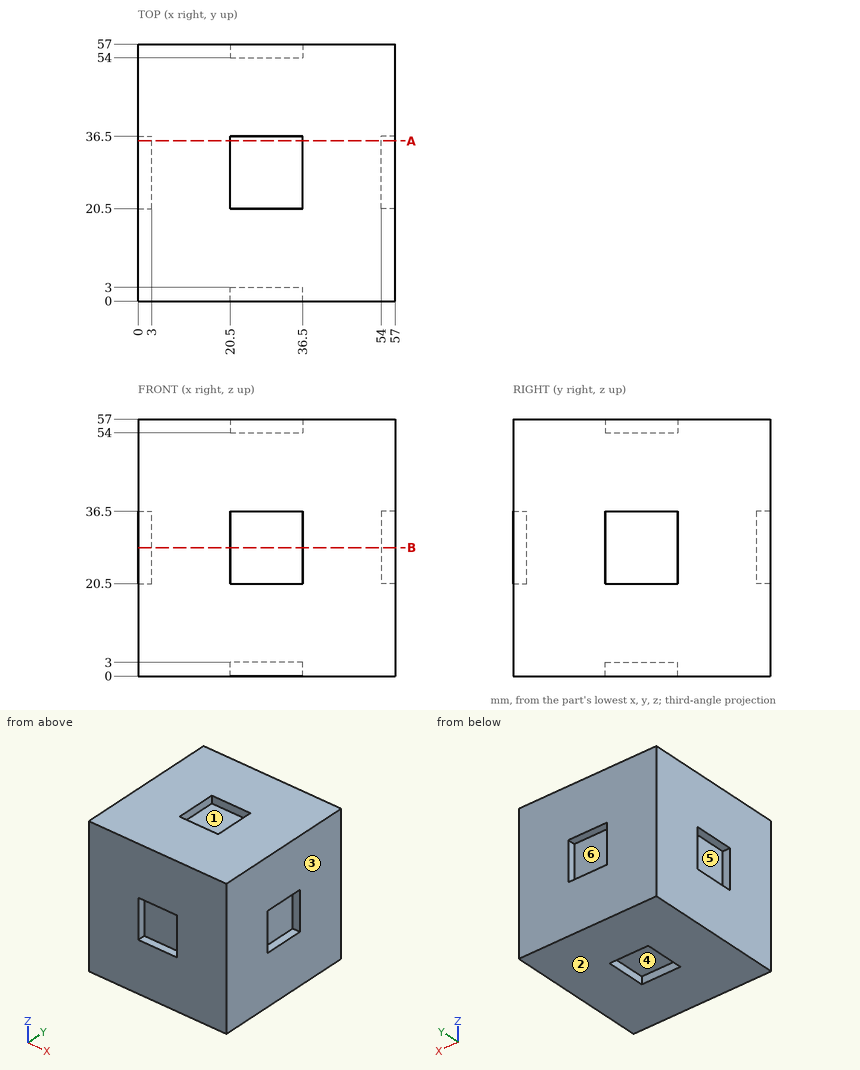
For this review, use the dimensioned drawing (mm, ordinates from the lowest corner) and the shaded views. A direction names the side the tool comes from. Coordinates: 2 decimals unless noted, no trailing zeros. Write each loop counter-clockwise with the first axis right and the second up, starting at its lowest first coordinate (ties: lowest second). Pieces come first, ordered by that corner, then holes. Notation, with made-up numbers: (44, 17) - (66, 17) arc R19 cw to (66, 27) - close; hole circle Ø11 at (-27, -9.75). An arc over 180 degrees is marked (long way). Answer in a Markdown table with one row per item. Add a question column.
Q1. Consider section A-A on y = 35.5. Give the boundary of the cut face in (x, z), then the cut area to 3 significant figures.
Q2. Draft analysis for pull direction X (two halves, no side actions). For the marked faces 1, 2 and 3, state which applies: +X half, -X half, draft (parallel to the pull), parting line (faces both ways), or undercut.
Q3. To check wall thickness, follow line 1 along Z through (x, y) = (22, 32.5). State the ranges of the line that lie inside material, in increasing order. Write a range as from..to.
Q4. Clearance check with flat-ended pins moving along their axes: pin 1 (6 mm diameter, centred on y = 32.5, z = 24.5, fed in from -X); pin 2 (13 mm diameter, centred on x = 29, y = 27.5, fed in from +Z); pin 3 (5 mm diameter, centred on x = 28.5, y = 29.5, fed in from -Z). State where each tip first meets the part, or that it passes through.
Q5. For the marked faces 4, 5 and 6, list the 3-axis set-ups (+Z, -Z, +X, -X, +Y, -Y) from which the entire face can be reached by the end or side of a thin tool; tool diameter is ignored.
Answers below:
| question | item | result |
|---|---|---|
| 1 | outline | (0, 0) - (20.5, 0) - (20.5, 3) - (36.5, 3) - (36.5, 0) - (57, 0) - (57, 20.5) - (54, 20.5) - (54, 36.5) - (57, 36.5) - (57, 57) - (36.5, 57) - (36.5, 54) - (20.5, 54) - (20.5, 57) - (0, 57) - (0, 36.5) - (3, 36.5) - (3, 20.5) - (0, 20.5) - close |
| 1 | area | 3,060 mm² |
| 2 | face 1 | undercut |
| 2 | face 2 | draft |
| 2 | face 3 | +X half |
| 3 | line 1 | 3..54 |
| 4 | pin 1 | x = 3 |
| 4 | pin 2 | z = 54 |
| 4 | pin 3 | z = 3 |
| 5 | face 4 | -Z |
| 5 | face 5 | -X |
| 5 | face 6 | +Y |
